Here's how the part is built. I have some questions about the finished solid (model axes, mm). Face numbers are marked on the shaded views. A direction names the side the tool comes from. Round coordinates to 2 decimals unless told otherwise and drop trailing zeros. Write each loop counter-clockwise with the first axis right and the second up, starting at its lowest first coordinate (ties: lowest second). Pieces come first, ordered by that corner, then holes. Notation, with made-up numbers: M -36.5,83 L -26.5,83 A16 cw -26.5,98 Z; hole C 2,21.5 d11. An arc over 180 degrees is marked long. Use one line per item in the form item = value. Start each with the question number.
Q1. I want a section at A-A on z = 0. List the corners of the cut face in (x, y) for me, and give its area (3 significant figures).
Q2. I'm going to push flat-ended pins straight in: pin 1 Ø3 at (y, z) = (73.5, 14.5) entering from +X; pin 2 Ø4 at (y, z) = (9.5, -48) entering from +X; pin 3 Ø8 at (x, y) = (-41.5, 111.5) entering from +Z; pin 4 Ø21 at (x, z) = (-73.5, -10.5) entering from -Y. Where does each tip first touch, or does it pass through?
Q3. I want a section at D-D on z = 66. List the corners of the cut face in (x, y) for me, and give its area (3 significant figures).
Q4. I need wall thicknesses on line 1 along Y through (x, z) = (-67, 19); line 2 along Y through (x, z) = (9, -6); line 3 along X through (y, z) = (28, -64.5). Which ranges of each line are inside material? Lowest first, please. Write a range as from..to.
Q5. For the marked faces 4, 5 and 6, which set-ups out of +Z, -Z, +X, -X, +Y, -Y let a thin tool reach every point of the face, with its end or its side?
Q6. We'd pull the mould along X, two halves only. Please class the marked faces 1, 2 and 3: +X half, -X half, draft (parallel to the pull), parting line (faces both ways), or undercut.
Q7. I want a section at B-B on x = -56. List the corners of the cut face in (y, z) for me, and give its area (3 significant figures).
Q8. I want a section at C-C on x = -37.5. List the corners of the cut face in (y, z) for me, and give its area (3 significant figures).
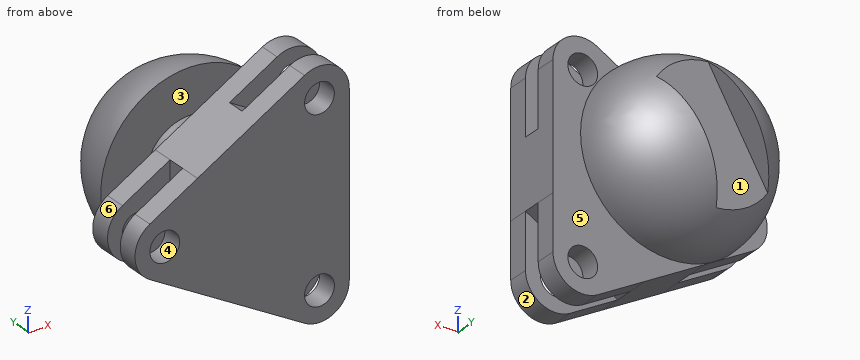
Autodesk Inventor part; units mm, degrees
ref_plane "Work Plane1" through (0, 70, 0) normal (0, 1, 0) x (1, 0, 0)
ref_plane "YZ Plane" through (0, 0, 0) normal (1, 0, 0) x (0, 1, 0)
ref_plane "XZ Plane" through (0, 0, 0) normal (0, 1, 0) x (-1, 0, 0)
sketch "Sketch1" plane through (0, 0, 0) normal (0, 1, 0) x (-1, 0, 0)
  line L0 (79.282, -17.3205) -> (-24.641, -77.3205)
  line L1 (-54.641, -60) -> (-54.641, 60)
  line L2 (-24.641, 77.3205) -> (79.282, 17.3205)
  arc A0 (79.282, -17.3205) -> (79.282, 17.3205) centre (69.282, 0) ccw
  arc A1 (-54.641, -60) -> (-24.641, -77.3205) centre (-34.641, -60) ccw
  arc A2 (-24.641, 77.3205) -> (-54.641, 60) centre (-34.641, 60) ccw
  line L3 (47.282, -35.7957) -> (47.282, 35.7957)
  line L4 (7.359, 58.8453) -> (-54.641, 23.0496)
  line L5 (-54.641, -23.0496) -> (7.359, -58.8453)
  circle A3 centre (69.282, 0) radius 10
  circle A4 centre (-34.641, -60) radius 10
  circle A5 centre (-34.641, 60) radius 10
  point P0 (0, 0)
  point P1 (109.282, 0)
  point P2 (-54.641, -94.641)
  point P3 (-54.641, 94.641)
  point P4 (0, 0)
  dimension "d18" = 20
  dimension "d19" = 120
  dimension "d22" = 22
  dimension "d25" = 360
  dimension "d27" = 20
extrude "Extrusion1" add sketch "Sketch1" along normal blind 40 contours L0 L5 L1 L4 L2 L3
extrude "Extrusion2" add sketch "Sketch1" along normal blind 14 contours L4 L1 A2 L2
extrude "Extrusion3" add sketch "Sketch1" against normal blind 14 from surface at 40 contours L4 L1 A2 L2
pattern_circular "Circular Pattern1" count 3 over 360 about axis through (0, -10, 0) along (0, 1, 0) of "Extrusion3", "Extrusion2"
ref_plane "Work Plane1" through (0, 70, 0) normal (0, 1, 0) x (1, 0, 0)
sketch "Sketch2" plane through (0, 70, 0) normal (0, 1, 0) x (1, 0, 0)
  line L0 (54.641, 60) -> (54.641, -60)
  line L1 (-79.282, 17.3205) -> (24.641, 77.3205)
  line L2 (24.641, -77.3205) -> (-79.282, -17.3205)
  circle A0 centre (-2.6063, 0) radius 57.2473
  circle A1 centre (-2.6063, 0) radius 30
  point P0 (0, 0)
  point P1 (-7.359, 58.8453)
  point P2 (-47.282, 35.7957)
  point P3 (-47.282, -35.7957)
  point P4 (-7.359, -58.8453)
  dimension "d38" = 60
extrude "Extrusion4" add sketch "Sketch2" against normal up to surface (30 mm away) contours A1
sketch "Sketch3" plane through (0, 0, 0) normal (0, 0, 1) x (1, 0, 0)
  line L0 (27.3937, 70) -> (-32.6063, 70)
  line L1 (57.3937, 70) -> (-2.6063, 70)
  line L2 (-2.6063, 70) -> (-2.6063, 130)
  arc A0 (57.3937, 70) -> (-2.6063, 130) centre (-2.6063, 70) ccw
  line L3 (-32.6063, 40) -> (27.3937, 40)
  point P0 (0, 0)
  point P1 (-2.6063, 70)
  dimension "d41" = 60
revolve "Revolution1" add sketch "Sketch3" angle 360 about axis through (-2.6063, 70, 0) along (0, 1, 0)
sketch "Sketch4" plane through (-79.282, 0, -17.3205) normal (-0.5, 0, -0.8660254) x (-0.8660254, 0, 0.5)
  arc A0 (2.2571, 70) -> (-117.7429, 70) centre (-57.7429, 70) ccw
  line L0 (-77.7429, 126.5685) -> (-77.7429, 110)
  line L1 (-77.7429, 110) -> (-37.7429, 110)
  line L2 (-37.7429, 110) -> (-37.7429, 126.5685)
  line L3 (2.2571, 70) -> (-117.7429, 70)
  point P0 (-60, 0)
  dimension "d43" = 40
  dimension "d44" = 40
extrude "Extrusion5" cut sketch "Sketch4" against normal up to surface contours L2 L1 L0 A0
properties part number "b4"
Reported:
q1.outline = M -89.28,0 L -79.28,0 L -79.28,14 L -89.28,14 Z; M -89.28,26 L -79.28,26 L -79.28,40 L -89.28,40 Z; M -62.61,70 L -32.61,70 L -32.61,40 L -59.28,40 L -59.28,26 L -47.28,26 L -47.28,14 L -59.28,14 L -59.28,0 L 54.64,0 L 54.64,40 L 27.39,40 L 27.39,70 L 57.39,70 A60 ccw 20.49,125.38 L 20.49,110 L -25.7,110 L -25.7,125.38 A60 ccw Z
q1.area = 11,300 mm^2
q2.pin_1 = 55.87
q2.pin_2 = 54.64
q2.pin_3 = 28.36
q2.pin_4 = 0
q3.outline = M 5.03,0 L 26.64,0 L 26.64,14 L 5.03,14 Z; M 5.03,26 L 26.64,26 L 26.64,40 L 5.03,40 Z; M 42.64,0 L 53.72,0 L 53.72,14 L 42.64,14 Z; M 42.64,26 L 53.72,26 L 53.72,40 L 42.64,40 Z
q3.area = 915 mm^2
q4.line_1 = 0..14, 26..40
q4.line_2 = 0..110
q4.line_3 = 2.44..25.71, 43.57..54.13
q5.face_4 = -Y
q5.face_5 = none
q5.face_6 = -X, +Y, -Y
q6.face_1 = undercut
q6.face_2 = parting line
q6.face_3 = draft
q7.outline = M 0,-30.76 L 14,-30.76 L 14,30.76 L 0,30.76 Z; M 26,-30.76 L 40,-30.76 L 40,30.76 L 26,30.76 Z; M 70,-27.37 A27.37 ccw 70,27.37 Z
q7.area = 2,900 mm^2
q8.outline = M 0,-41.44 L 40,-41.44 L 40,41.44 L 0,41.44 Z; M 70,-48.81 A48.81 ccw 110,-27.97 L 110,-20.44 L 114.33,-20.44 A48.81 ccw 70,48.81 Z
q8.area = 7,040 mm^2
